from build123d import *

# Parameters (mm, degrees)
F0_W      = 45
F0_H      = 12
F0_R      = 2.2
F1_DEPTH  = 16.8
F3_DEPTH  = 12.001
F4_R      = 8.1
F5_DEPTH  = 3.05
F6_R      = 8.1
F7_DEPTH  = 3.05
F8_R      = 4.5
F8_R_2    = 2.2
F9_DEPTH  = 9
F10_SIZE  = 2.29999
F11_R     = 2
F12_W     = 12
F12_H     = 12
F12_R     = 1.85
F13_DEPTH = 4
F14_R     = 4


# Not quite as in the source:
# - a fillet or chamfer is up to 0.001 mm smaller than in the source, because OpenCascade refuses the exact size


with BuildPart() as f1:
    # F0 (on Top) → F1 (new body)
    with BuildSketch(Plane.XY):
        Rectangle(F0_W, F0_H)
        with Locations((-13, 0)):
            Circle(F0_R, mode=Mode.SUBTRACT)
        with Locations((13, 0)):
            Circle(F0_R, mode=Mode.SUBTRACT)
    extrude(amount=F1_DEPTH)

    # F2 (on face) → F3 (cut, through all)
    with BuildSketch(Plane(origin=(0, 6, 0), x_dir=(-1, 0, 0), z_dir=(0, 1, 0))):
        with BuildLine():
            ThreePointArc((-6.0794736614, 16.8), (0, 11.2), (6.0794736614, 16.8))
            Line((6.0794736614, 16.8), (-6.0794736614, 16.8))
        make_face()
        with BuildLine():
            Line((-6.0794736614, 16.8), (6.0794736614, 16.8))
            ThreePointArc((6.0794736614, 16.8), (6.0948662551, 17.0497894234), (6.1, 17.3))
            ThreePointArc((6.1, 17.3), (-0.2502105766, 23.3948662551), (-6.0794736614, 16.8))
        make_face()
    extrude(amount=-F3_DEPTH, mode=Mode.SUBTRACT)

    # F4 (on face) → F5 (cut)
    with BuildSketch(Plane(origin=(0, 6, 0), x_dir=(-1, 0, 0), z_dir=(0, 1, 0))):
        with Locations((0, 17.3)):
            Circle(F4_R)
    extrude(amount=-F5_DEPTH, mode=Mode.SUBTRACT)

    # F6 (on face) → F7 (cut)
    with BuildSketch(Plane.XZ.offset(6)):
        with Locations((0, 17.3)):
            Circle(F6_R)
    extrude(amount=-F7_DEPTH, mode=Mode.SUBTRACT)

    # F8 (on face) → F9 (cut)
    with BuildSketch(Plane(origin=(0, 0, 0), x_dir=(1, 0, 0), z_dir=(0, 0, -1))):
        with Locations((-13, 0)):
            Circle(F8_R)
        with Locations((-13, 0)):
            Circle(F8_R_2, mode=Mode.SUBTRACT)
        with Locations((13, 0)):
            Circle(F8_R)
        with Locations((13, 0)):
            Circle(F8_R_2, mode=Mode.SUBTRACT)
    extrude(amount=-F9_DEPTH, mode=Mode.SUBTRACT)

    # F10 (size 2.3 in the source; OpenCascade refuses exactly that, so slightly less here)
    f10_edges = [f1.edges().sort_by_distance(p)[0] for p in [
        (-17.5, 0, 9),
        (8.5, 0, 9),
    ]]
    chamfer(f10_edges, length=F10_SIZE)

    # F11
    f11_edges = [f1.edges().sort_by_distance(p)[0] for p in [
        (22.5, -6, 8.4),
        (-22.5, -6, 8.4),
        (22.5, 6, 8.4),
        (-22.5, 6, 8.4),
    ]]
    fillet(f11_edges, radius=F11_R)

    # F12 (on face) → F13 (join)
    with BuildSketch(Plane.XY.offset(16.8)):
        with Locations((26.5, 0)):
            Rectangle(F12_W, F12_H)
        with Locations((28.5, 0)):
            Circle(F12_R, mode=Mode.SUBTRACT)
    extrude(amount=-F13_DEPTH)

    # F14
    f14_edges = [f1.edges().sort_by_distance(p)[0] for p in [
        (32.5, -6, 14.8),
        (32.5, 6, 14.8),
    ]]
    fillet(f14_edges, radius=F14_R)


solid = f1.part
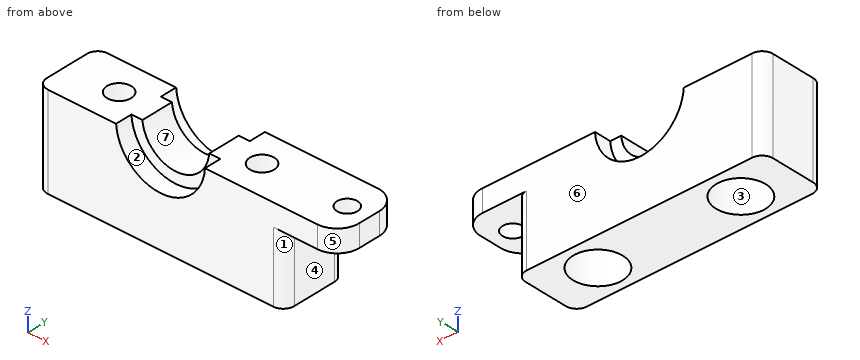
Model file for the job. Use its own axes, mm. Face numbers are marked on the shaded views. A direction names the side the tool comes from. Coordinates: 2 decimals unless noted, no trailing zeros. Write each loop counter-clockwise with the first axis right and the second up, starting at its lowest first coordinate (ties: lowest second). Pieces come first, ordered by that corner, then holes. Notation, with made-up numbers: (-33.75, 27.5) - (8.25, 27.5) arc R32 cw to (8.25, 65.5) - close; hole circle Ø5 at (45.5, 9). An arc over 180 degrees is marked (long way). Write each question's results on one line, items separated by ' | '. Start each with the question number.
1) 3-axis set-ups, long thin cutter, end or side, ignore diameter. For the marked faces 1, 2, 3 and 4: which of +Z, -Z, +X, -X, +Y, -Y reach the whole face in a straight line?
2) Cut at D-D (x = 3.5). Write the cut outline in (y, z).
3) Cut at C-C (z = 4.25). Write the cut outline in (x, y).
4) Mould opens along X. For the marked faces 5, 6 and 7 say: pulls with the +X half, pulls with the -X half, needs draft (parallel to the pull), parting line crosses it, or undercut.
5) Flat gauge pins, fed straight in: P1, Ø1, axis at x = -9, y = 3, coming from the -Z side; P2, Ø2, axis at x = 12, y = -0.5, coming from the -Z side; P3, Ø6, axis at y = 0.5, z = 9, coming from the +X side; P4, Ø2, axis at x = 3, z = 12, coming from the +Y side. Where does each tip first touch, or does it go through?
6) Cut at B-B (y = 0). Count the separate pieces of the cut face and the enclosed holes in it, then the cut area to 3 significant figures.
7) Probe line 1 along X through (y, z) = (0, 3); line 2 along X through (y, z) = (-1, 13); line 3 along X through (y, z) = (-1.75, 6.5). List the from-to ranges inside material, lowest first. Write a range as from..to.
Returned:
1) face 1: -Z, +X, -Y | face 2: +Z, -Y | face 3: -Z | face 4: -Z, +X, +Y, -Y
2) outline: (-6, 0) - (6, 0) - (6, 10) - (2.95, 10) - (2.95, 12.3) - (-2.95, 12.3) - (-2.95, 10) - (-6, 10) - close
3) outline: (-22.5, -4) arc R2 ccw to (-20.5, -6) - (20.5, -6) arc R2 ccw to (22.5, -4) - (22.5, 4) arc R2 ccw to (20.5, 6) - (-20.5, 6) arc R2 ccw to (-22.5, 4) - close; hole circle Ø9 at (-13, 0); hole circle Ø9 at (13, 0)
4) face 5: pulls with the +X half | face 6: needs draft | face 7: undercut
5) P1: z = 0 | P2: through | P3: x = 22.5 | P4: y = 2.95
6) separate pieces: 4 | enclosed holes: 0 | area: 509 mm^2
7) line 1: -22.5..-17.5, -8.5..8.5, 17.5..22.5 | line 2: -22.5..-14.96, -11.04..-4.33, 4.33..11.04, 14.96..26.94, 30.06..32.5 | line 3: -22.5..-17.15, -8.85..8.85, 17.15..22.5
